from build123d import *

# Parameters (mm, degrees)
F1_DEPTH             = 7.5
F2_R                 = 7.49999
F3_R                 = 3
F6_D                 = 4.5
F6_CSINK_D           = 6.5
F6_CSINK_ANGLE       = 90
F6_ON_F5_D           = 4.5
F6_ON_F5_CSINK_D     = 6.5
F6_ON_F5_CSINK_ANGLE = 90


# Not quite as in the source:
# - a fillet or chamfer is up to 0.001 mm smaller than in the source, because OpenCascade refuses the exact size


with BuildPart() as f1:
    # F0 (on Front) → F1 (new body, symmetric)
    with BuildSketch(Plane.XZ):
        Polygon((0, 0), (0, -32.5), (2, -32.5), (2, -2), (32.5, -2), (32.5, 0), align=None)
    extrude(amount=F1_DEPTH, both=True)

    # F2 (radius 7.5 in the source; OpenCascade refuses exactly that, so slightly less here)
    f2_edges = [f1.edges().sort_by_distance(p)[0] for p in [
        (32.5, -7.5, -1),
        (32.5, 7.5, -1),
        (1, -7.5, -32.5),
        (1, 7.5, -32.5),
    ]]
    fillet(f2_edges, radius=F2_R)

    # F3
    f3_edges = [f1.edges().sort_by_distance(p)[0] for p in [
        (2, 0, -2),
        (0, 0, 0),
    ]]
    fillet(f3_edges, radius=F3_R)

    # F6 (through all)
    with Locations(Plane(origin=(0, 0, -2), x_dir=(1, 0, 0), z_dir=(0, 0, -1))):
        with Locations((12.8, 0), (25.5, 0)):
            CounterSinkHole(F6_D / 2, F6_CSINK_D / 2, counter_sink_angle=F6_CSINK_ANGLE)

    # F6 on F5 (through all)
    with Locations(Plane.YZ.offset(2)):
        with Locations((0, -25.5), (0, -12.8)):
            CounterSinkHole(F6_ON_F5_D / 2, F6_ON_F5_CSINK_D / 2, counter_sink_angle=F6_ON_F5_CSINK_ANGLE)


solid = f1.part
Check sheet for the modelled part. Datum: model origin and axes. Units: mm. A direction names the side the tool comes from. Round coordinates to 2 decimals unless told otherwise and drop trailing zeros. Order: outer loops, then holes, each group sorted by start corner. A loop starts at its lowest first (then second) coordinate and runs counter-clockwise, first axis right, second up.
(1) Cross-section at B-B, the plane x = 12.8. Enter the section's corners in (y, z), and give its area (3 significant figures).
(2) Go/stop test with flat-tipped pins: P1, Ø5, axis at x = 26.5, y = 6, coming from the -Z side; P2, Ø7.5, axis at y = 2.5, z = -20, coming from the +X side. Record where each tip stops, or that it passes through.
(3) Access from +Z, -Z, +X, -X, +Y, -Y to the whole of each face (thin tool, end or side, straight path). Record for faces 1 (the cylindrical face through (1.014, -5.361, -30.245)), 2 (the flat face through (19, 0, -2)).
(4) Cross-section at C-C, the plane y = -6. Enter the section's corners in (x, z), and give its area (3 significant figures).
(5) Scan lines: probe 1 along X at (y, z) = (-2.25, -22); probe 2 along Z at (x, y) = (12, -4.25); probe 3 along Y at (x, z) = (12.8, -0.75). Record each from-to range of solid material in increasing order.
(6) Cross-section at A-A, the plane z = -12.8. Enter the section's corners in (x, y).
(7) Draft check along X on faces 3 (the flat face through (0, 0, -18)), 4 (the flat face through (1, -7.5, -8)), 5 (the cylindrical face through (14.46, -1.52, -0.49)). Enter one of: pulls with the +X half, pulls with the -X half, needs draft (parallel to the pull), parting line crosses it, or undercut.
(8) Cross-section at D-D, the plane x = 9. Enter the section's corners in (y, z).
Check sheet entries:
1. outline: (-7.5, -2) - (-3.25, -2) - (-2.25, -1) - (-2.25, 0) - (-7.5, 0) - close; (2.25, -1) - (3.25, -2) - (7.5, -2) - (7.5, 0) - (2.25, 0) - close
1. area: 20.0 mm2
2. P1: stops at z = -2
2. P2: stops at x = 2
3. face 1: -Z, +X, -X, -Y
3. face 2: -Z, +X, +Y, -Y
4. outline: (0, -29.5) - (2, -29.5) - (2, -5) arc R3 cw to (5, -2) - (29.5, -2) - (29.5, 0) - (3, 0) arc R3 ccw to (0, -3) - close
4. area: 114 mm2
5. probe 1: x = 0 to 2
5. probe 2: z = -2 to 0
5. probe 3: y = -7.5 to -2.25, 2.25 to 7.5
6. outline: (0, -7.5) - (2, -7.5) - (2, -3.25) - (1, -2.25) - (0, -2.25) - close; (0, 2.25) - (1, 2.25) - (2, 3.25) - (2, 7.5) - (0, 7.5) - close
7. face 3: pulls with the -X half
7. face 4: needs draft
7. face 5: undercut
8. outline: (-7.5, -2) - (7.5, -2) - (7.5, 0) - (-7.5, 0) - close
